Autodesk Inventor part; units mm, degrees
ref_plane "YZ Plane" through (0, 0, 0) normal (1, 0, 0) x (0, 1, 0)
ref_plane "XZ Plane" through (0, 0, 0) normal (0, 1, 0) x (-1, 0, 0)
ref_plane "XY Plane" through (0, 0, 0) normal (0, 0, 1) x (1, 0, 0)
sketch "Sketch1" plane through (0, 0, 0) normal (0, 0, 1) x (1, 0, 0)
  line L0 (0, 0) -> (296.3316, 0)
  line L1 (296.3316, 0) -> (296.3316, -355.6)
  line L2 (296.3316, -355.6) -> (0, -355.6)
  line L3 (0, -355.6) -> (0, 0)
  dimension "d0" = 296.3316
  dimension "d1" = 355.6
extrude "Extrusion1" add sketch "Sketch1" along normal blind 6.35
sketch "Sketch2" plane through (0, 0, 0) normal (0, 1, 0) x (1, 0, 0)
  line L0 (296.3316, -6.35) -> (0, -6.35)
  line L1 (0, -6.35) -> (-3.6662, -6.35)
  line L2 (-3.6662, -6.35) -> (0, 0)
  line L3 (0, 0) -> (0, -6.35)
  line L4 (0, 0) -> (0, -6.35)
  line L5 (0, -6.35) -> (0, 0)
  line L6 (296.3316, -6.35) -> (299.9978, -6.35)
  line L7 (296.3316, 0) -> (296.3316, -6.35)
  line L8 (299.9978, -6.35) -> (296.3316, 0)
  line L9 (296.3316, 0) -> (296.3316, -6.35)
  dimension "d4" = 30
  dimension "d5" = 60
extrude "Extrusion2" add sketch "Sketch2" against normal blind 355.6
sketch "Sketch5" plane through (0, 0, 6.35) normal (0, 0, 1) x (1, 0, 0)
  line L0 (139.1658, -100) -> (157.1658, -100)
  line L1 (157.1658, -100) -> (157.1658, -110)
  line L2 (157.1658, -110) -> (139.1658, -110)
  line L3 (139.1658, -110) -> (139.1658, -100)
  line L4 (-3.6662, 0) -> (299.9978, 0)
  point P0 (0, 0)
  point P1 (148.1658, -100)
  point P2 (148.1658, 0)
  dimension "d77" = 18
  dimension "d78" = 10
  dimension "d79" = 100
extrude "Extrusion5" cut sketch "Sketch5" against normal through all
properties part number "BA03" material "ABS Plastic"
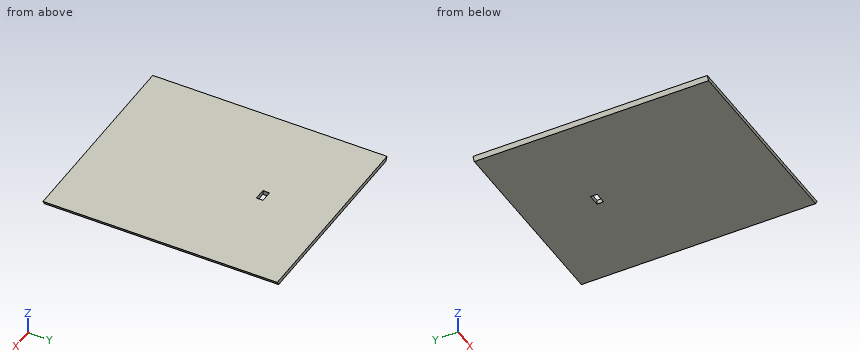
Source: CAD feature listing. Evaluate the final solid. Frame: model axes, mm. Round coordinates to 2 decimals unless told otherwise and drop trailing zeros. Loops run counter-clockwise (first coordinate to the right, second up) from the corner with the lowest first, then second, coordinate; pieces in that order, holes last.
Q1. First-contact query: P1, Ø3, axis at y = -105.5, z = 2, coming from the +X side; P2, Ø1.5, axis at y = -107.5, z = 4.5, coming from the -X side; P3, Ø1, axis at y = -263, z = 4, coming from the +X side. Flat tips, straight axial feed; report the tip coordinate or a pass-through.
Q2. Section A-A, the plane x = 153. Return loops of the section in (y, z), plus the area to 3 significant figures.
Q3. Ray query, line 1 (X direction, y = -138, z = 6); line 2 (X direction, y = -213, z = 2.25). Return the intervals inside material, ascending.
Q4. Section B-B, the plane z = 2.75. Return loops of the section in (x, y), plus the area to 3 significant figures.
Solutions:
1. P1: stops at x = 298.35
1. P2: stops at x = -3.03
1. P3: stops at x = 298.93
2. outline: (-355.6, 0) - (-110, 0) - (-110, 6.35) - (-355.6, 6.35) - close; (-100, 0) - (0, 0) - (0, 6.35) - (-100, 6.35) - close
2. area: 2,190 mm2
3. line 1: x = -3.46 to 299.8
3. line 2: x = -1.3 to 297.63
4. outline: (-1.59, -355.6) - (297.92, -355.6) - (297.92, 0) - (-1.59, 0) - close; hole (139.17, -110) - (157.17, -110) - (157.17, -100) - (139.17, -100) - close
4. area: 106,000 mm2
